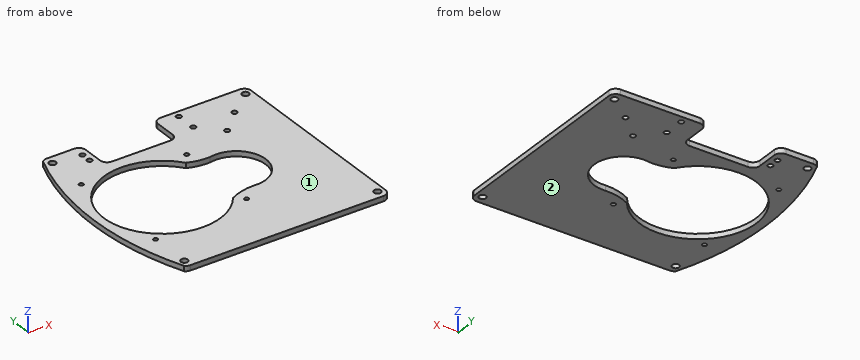
Autodesk Inventor part; units mm, degrees
ref_plane "YZ Plane" through (0, 0, 0) normal (1, 0, 0) x (0, 1, 0)
ref_plane "XZ Plane" through (0, 0, 0) normal (0, 1, 0) x (-1, 0, 0)
ref_plane "XY Plane" through (0, 0, 0) normal (0, 0, 1) x (1, 0, 0)
sketch "Эскиз1" plane through (0, 0, 0) normal (0, 0, 1) x (1, 0, 0)
  line L0 (0, 29) -> (0, -30)
  circle A0 centre (35, 25) radius 1.25
  circle A1 centre (-22, 31) radius 1.25
  circle A2 centre (-22, -31) radius 1.25
  circle A3 centre (35, -25) radius 1.25
  arc A4 (45.1579, -16.824) -> (42.7931, 16.7046) centre (46.5307, 0.1205) ccw
  line L1 (35, -25) -> (0, -25)
  circle A5 centre (-22, -55) radius 2
  circle A6 centre (90, -55) radius 2
  circle A7 centre (90, 55) radius 2
  circle A8 centre (-22, 55) radius 2
  line L2 (-22, -60) -> (90, -60)
  line L3 (94, -56) -> (94, 56)
  arc A9 (94, 56) -> (90, 60) centre (90, 56) ccw
  arc A10 (90, -60) -> (94, -56) centre (90, -56) ccw
  arc A11 (-24.8284, -58.8284) -> (-22, -60) centre (-22, -56) ccw
  arc A12 (-22, 60) -> (-24.8284, 58.8284) centre (-22, 56) ccw
  line L4 (94, 0) -> (94, 6)
  circle A13 centre (52, 44) radius 1.5
  circle A14 centre (52, 56) radius 1.5
  line L5 (-22, 60) -> (-6, 60)
  line L6 (44, 60) -> (90, 60)
  arc A15 (46.5295, -16.8795) -> (30.2933, -20.5081) centre (44.6409, -46.5678) ccw
  arc A16 (30.2933, 18.9458) -> (42.7931, 16.7046) centre (41.489, 45.4087) ccw
  line L7 (36, 40) -> (2, 40)
  line L8 (-2, 44) -> (-2, 56)
  line L9 (40, 56) -> (40, 44)
  arc A17 (44, 60) -> (40, 56) centre (44, 56) ccw
  arc A18 (36, 40) -> (40, 44) centre (36, 44) ccw
  arc A19 (-2, 44) -> (2, 40) centre (2, 44) ccw
  arc A20 (-2, 56) -> (-6, 60) centre (-6, 56) ccw
  circle A21 centre (-6, 53) radius 1.5
  circle A22 centre (-6, 47) radius 1.5
  arc A23 (-24.8284, 58.8284) -> (-24.8284, -58.8284) centre (124.4782, 0) ccw
  circle A24 centre (63.4885, 32.25) radius 1.5
  circle A25 centre (76, 44) radius 1.5
  arc A26 (30.2933, 18.9458) -> (30.2933, -20.5081) centre (2.8162, -0.7812) ccw
  point P0 (0, 0)
  point P1 (-26, -60)
  point P2 (94, -60)
  dimension "d3" = 2.5
  dimension "d4" = 2.5
  dimension "d5" = 2.5
  dimension "d6" = 2.5
  dimension "d10" = 50
  dimension "d11" = 34
  dimension "d39" = 4
  dimension "d44" = 120
  dimension "d46" = 4
  dimension "d70" = 4
  dimension "d71" = 3
  dimension "d72" = 3
  dimension "d75" = 3
  dimension "d76" = 3
extrude "Выдавливание4" add sketch "Эскиз1" along normal blind 3
properties part number "06-01-Платформа для лидара"
Geometry: final body of the model. Coordinates: model frame, mm. Face numbers are marked on the shaded views. Coordinates: 2 decimals unless noted, no trailing zeros. Loops run counter-clockwise (first coordinate to the right, second up) from the corner with the lowest first, then second, coordinate; pieces in that order, holes last. Notation, with made-up numbers: (-21, -36.75) - (-6, -36.75) arc R10 cw to (-6, -24.75) - close; hole circle Ø11 at (61, 24). An arc over 180 degrees is marked (long way). One line per question, with ' | ' between items. Start each with the question number.
(1) Cut plane B-B on x = 52. Output: boundary loops of the cut face in (y, z).
(2) Ray query, L1, parallel to Y at x = 90, z = 1.9; L2, parallel to Y at x = 35, z = 1.4; L3, parallel to Y at x = 52, z = 0.75. Return the intervals inside material, ascending. Write a range as from..to.
(3) Cut plane A-A on x = 76. Output: boundary loops of the cut face in (y, z), and give its area (3 significant figures).
(4) Cut plane D-D on z = 2.05. Count the separate pieces of the cut face and the enclosed holes in it, and give its area (3 significant figures).
(5) Cut plane C-C on y = 47. Output: boundary loops of the cut face in (x, z), and give its area (3 significant figures).
(6) Draft query along Z for the marked faces 1 and 2. Return one class per face: +Z half, -Z half, draft (parallel to the pull), parting line (faces both ways), or undercut.
(7) First-contact query: pin 1 (0.9 mm diameter, centred on x = 25.5, z = 1, fed in from +Y). Flat tip, straight axial feed; report the tip coordinate or a pass-through.
Here are the results:
1) outline: (-60, 0) - (-15.98, 0) - (-15.98, 3) - (-60, 3) - close; (16.22, 0) - (42.5, 0) - (42.5, 3) - (16.22, 3) - close; (45.5, 0) - (54.5, 0) - (54.5, 3) - (45.5, 3) - close; (57.5, 0) - (60, 0) - (60, 3) - (57.5, 3) - close
2) L1: -60..-57, -53..53, 57..60 | L2: -60..-26.25, -23.75..-18.43, 17.42..23.75, 26.25..40 | L3: -60..-15.98, 16.22..42.5, 45.5..54.5, 57.5..60
3) outline: (-60, 0) - (42.5, 0) - (42.5, 3) - (-60, 3) - close; (45.5, 0) - (60, 0) - (60, 3) - (45.5, 3) - close | area: 351 mm²
4) separate pieces: 1 | enclosed holes: 15 | area: 9,730 mm²
5) outline: (-28.96, 0) - (-7.5, 0) - (-7.5, 3) - (-28.96, 3) - close; (-4.5, 0) - (-2, 0) - (-2, 3) - (-4.5, 3) - close; (40, 0) - (94, 0) - (94, 3) - (40, 3) - close | area: 234 mm²
6) face 1: +Z half | face 2: -Z half
7) pin 1: y = 40
